For this review, take the finished solid that the model builds, in its own axes (mm). Face numbers are marked on the shaded views. A direction names the side the tool comes from. Coordinates: 2 decimals unless noted, no trailing zeros. Loops run counter-clockwise (first coordinate to the right, second up) from the corner with the lowest first, then second, coordinate; pieces in that order, holes last. Notation, with made-up numbers: (18, 5) - (31, 5) arc R22 ccw to (31, 34) - close; hole circle Ø11 at (-6, 70.5). An arc over 180 degrees is marked (long way). One line per item, written item: value. Start each with the question number.
1. For the marked faces 4, 5 and 6, list the 3-axis set-ups (+Z, -Z, +X, -X, +Y, -Y) from which the entire face can be reached by the end or side of a thin tool; tool diameter is ignored.
2. Take a section at B-B, the plane z = 19. Count the separate pieces of the cut face and the enclosed holes in it, and give its area (3 significant figures).
3. Take a section at A-A, the plane x = 15. State the section outline as (y, z) points, and give its area (3 significant figures).
4. The part is to be moulded in two halves that separate along Z. For the marked faces 1, 2 and 3, say which applies: released by +Z, released by -Z, zero draft, split by the parting line, or undercut.
5. To check wall thickness, follow line 1 (Z direction, x = 18.5, y = -29.5); line 2 (Y direction, x = 25, z = 43.5); line 3 (X direction, y = -15.5, z = 22.5). State the ranges of each line that lie inside material, in increasing order. Write a range as from..to.
6. Take a section at C-C, the plane y = -40. State the section outline as (x, z) points.
7. Insertion check: pin 1 (10 mm diameter, centred on y = -5.5, z = 18, fed in from +X); pin 2 (19 mm diameter, centred on x = 31.21, z = 25.05, fed in from -Y); pin 3 (8 mm diameter, centred on y = -5.5, z = 47, fed in from +X). Each pin has a flat end and moves straight along its axis. Give the tip position at first contact, or say it passes through.
```python
from build123d import *

# Parameters (mm, degrees)
F1_DEPTH = 51.816
F2_DEPTH = 10.16
F3_R     = 8.94315
F4_DEPTH = 101.6
F5_R     = 9.219665
F6_DEPTH = 50.8
F7_R     = 10.48142
F8_DEPTH = 50.8
F9_R     = 5.08


with BuildPart() as f1:
    # F0 (on Front) → F1 (new body)
    with BuildSketch(Plane.XZ):
        Polygon((54.062217, 43.212991), (0, 43.212991), (0, 0), (87.161534, 0), align=None)
    extrude(amount=F1_DEPTH)

    # F0 (on Front) → F2 (join)
    with BuildSketch(Plane.XZ):
        Polygon((61.417621, 56.452714), (0, 56.452714), (0, 43.212991), (54.062217, 43.212991), (87.161534, 0), (107.756652, 0), align=None)
    extrude(amount=F2_DEPTH)

    # F3 (on Right) → F4 (cut)
    with BuildSketch(Plane.YZ):
        with Locations((-28.951842, 23.85469)):
            Circle(F3_R)
    extrude(amount=F4_DEPTH, mode=Mode.SUBTRACT)

    # F5 (on face) → F6 (cut)
    with BuildSketch(Plane.XZ.offset(51.816)):
        with Locations((32.87245, 25.28506)):
            Circle(F5_R)
    extrude(amount=F6_DEPTH, mode=Mode.SUBTRACT)

    # F7 (on face) → F8 (cut)
    with BuildSketch(Plane.XZ.offset(51.816)):
        with Locations((31.210523, 25.047641)):
            Circle(F7_R)
    extrude(amount=-F8_DEPTH, mode=Mode.SUBTRACT)

    # F9
    f9_edges = [f1.edges().sort_by_distance(p)[0] for p in [
        (30.70881, -10.16, 56.452714),
        (84.587136, -10.16, 28.226357),
        (27.031109, -51.816, 43.212991),
        (70.611876, -51.816, 21.606496),
    ]]
    fillet(f9_edges, radius=F9_R)


solid = f1.part
```
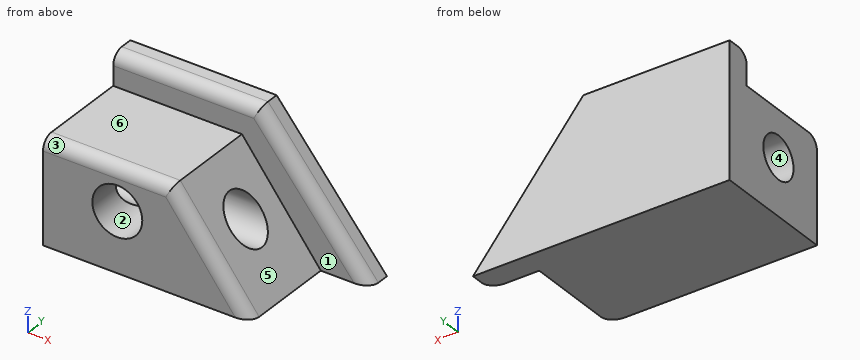
Solutions:
1. face 4: +X, -X
1. face 5: +Z, +X, -Y
1. face 6: +Z, +X, -X, -Y
2. separate pieces: 3
2. enclosed holes: 0
2. area: 2,240 mm2
3. outline: (-51.82, 0) - (0, 0) - (0, 56.45) - (-5.08, 56.45) arc R5.08 ccw to (-10.16, 51.37) - (-10.16, 43.21) - (-46.74, 43.21) arc R5.08 ccw to (-51.82, 38.13) - close; hole circle Ø17.89 at (-28.95, 23.85)
3. area: 2,110 mm2
4. face 1: zero draft
4. face 2: undercut
4. face 3: released by +Z
5. line 1: 0..14.93, 32.78..43.21
5. line 2: -10.16..0
5. line 3: 0..21.04, 41.38..69.93
6. outline: (0, 0) - (87.16, 0) - (54.06, 43.21) - (0, 43.21) - close; hole circle Ø20.96 at (31.21, 25.05)
7. pin 1: x = 97.08
7. pin 2: y = -1.02
7. pin 3: x = 72.45
